from build123d import *

# Parameters (mm, degrees)
BOSS_EXTRUDE1_DEPTH              = 5.334
FILLET1_R                        = 0.508
BOSS_EXTRUDE2_DEPTH              = 1.5875
F_56_0_0465_DIAMETER_HOLE1_D     = 1.1811
F_56_0_0465_DIAMETER_HOLE1_DEPTH = 5.08
CUT_EXTRUDE3_REACH               = 13.094
CUT_EXTRUDE3_START_RADIUS        = 21.519514579
CUT_EXTRUDE3_END_RADIUS          = 21.519514579
SKETCH9_W                        = 0.762
SKETCH9_H                        = 6.35


with BuildPart() as part:
    # Sketch1 → Boss-Extrude1 (new body)
    with BuildSketch(Plane.XY):
        with BuildLine():
            Line((3.301999954, 5.156199954), (-3.301999954, 5.156199954))
            ThreePointArc((-3.301999954, 5.156199954), (-4.613117348, 4.613117348), (-5.156199954, 3.301999954))
            Line((-5.156199954, 3.301999954), (-5.156199954, -3.301999954))
            ThreePointArc((-5.156199954, -3.301999954), (-4.613117348, -4.613117348), (-3.301999954, -5.156199954))
            Line((-3.301999954, -5.156199954), (3.301999954, -5.156199954))
            ThreePointArc((3.301999954, -5.156199954), (4.613117348, -4.613117348), (5.156199954, -3.301999954))
            Line((5.156199954, -3.301999954), (5.156199954, 3.301999954))
            ThreePointArc((5.156199954, 3.301999954), (4.613117348, 4.613117348), (3.301999954, 5.156199954))
        make_face()
    extrude(amount=-BOSS_EXTRUDE1_DEPTH)

    # Fillet1
    fillet1_edges = [part.edges().sort_by_distance(p)[0] for p in [
        (0, 5.156199954, 0),
        (4.613117348, 4.613117348, 0),
        (5.156199954, 0, 0),
        (4.613117348, -4.613117348, 0),
        (0, -5.156199954, 0),
        (-4.613117348, -4.613117348, 0),
        (-5.156199954, 0, 0),
        (-4.613117348, 4.613117348, 0),
    ]]
    fillet(fillet1_edges, radius=FILLET1_R)

    # Sketch4 → Boss-Extrude2 (add)
    with BuildSketch(Plane(origin=(0, 0, -5.334), x_dir=(-1, 0, 0), z_dir=(0, 0, -1))):
        with BuildLine():
            Line((-5.664199954, 3.301999954), (-5.664199954, -3.301999954))
            ThreePointArc((-5.664199954, -3.301999954), (-4.972327592, -4.972327592), (-3.301999954, -5.664199954))
            Line((-3.301999954, -5.664199954), (3.301999954, -5.664199954))
            ThreePointArc((3.301999954, -5.664199954), (4.972327592, -4.972327592), (5.664199954, -3.301999954))
            Line((5.664199954, -3.301999954), (5.664199954, 3.301999954))
            ThreePointArc((5.664199954, 3.301999954), (4.972327592, 4.972327592), (3.301999954, 5.664199954))
            Line((3.301999954, 5.664199954), (-3.301999954, 5.664199954))
            ThreePointArc((-3.301999954, 5.664199954), (-4.972327592, 4.972327592), (-5.664199954, 3.301999954))
        make_face()
    extrude(amount=BOSS_EXTRUDE2_DEPTH)

    # #56 (0.0465) Diameter Hole1
    with Locations(Plane(origin=(0, 0, -6.9215), x_dir=(-1, 0, 0), z_dir=(0, 0, -1))):
        with Locations((0, 0)):
            Hole(F_56_0_0465_DIAMETER_HOLE1_D / 2, depth=F_56_0_0465_DIAMETER_HOLE1_DEPTH)

    # Sketch8 → Cut-Revolve1 (revolve, cut)
    with BuildSketch(Plane(origin=(0, 0, 0), x_dir=(0, 0, -1), z_dir=(1, 0, 0)), mode=Mode.PRIVATE) as cut_revolve1_sk:
        with BuildLine():
            Line((0, 4.648199954), (0, 0))
            Line((0, 0), (0.508, 0))
            ThreePointArc((0.508, 0), (0.380623019, 2.337938558), (0, 4.648199954))
        make_face()
    revolve(cut_revolve1_sk.sketch.rotate(Axis((0, 0, -0.508), (0, 0, 1)), 90), axis=Axis((0, 0, -0.508), (0, 0, 1)), mode=Mode.SUBTRACT)

    # Cut-Extrude3: from a sphere face, 13.094 long prism both ways, kept between that surface and its translate by the depth
    cut_extrude3_start = Location((0, 0, 21.011514579)) * Sphere(CUT_EXTRUDE3_START_RADIUS, mode=Mode.PRIVATE)
    cut_extrude3_end = Location((0, 0, 20.503514579)) * Sphere(CUT_EXTRUDE3_END_RADIUS, mode=Mode.PRIVATE)
    # Sketch9 → Cut-Extrude3 (cut, from a surface)
    with BuildSketch(Plane.XY, mode=Mode.PRIVATE) as cut_extrude3_sk1:
        Rectangle(SKETCH9_W, SKETCH9_H)
    cut_extrude3_tool1 = extrude(cut_extrude3_sk1.sketch, amount=CUT_EXTRUDE3_REACH, both=True, mode=Mode.PRIVATE)
    add(((cut_extrude3_tool1 - cut_extrude3_start) & cut_extrude3_end).solids().sort_by_distance((0, 0, -0.52308))[0], mode=Mode.SUBTRACT)


solid = part.part
Input: part model. Units: mm. Frame: model coordinates. A direction names the side the tool comes from. Coordinates: 2 decimals unless noted, no trailing zeros. Loops run counter-clockwise (first coordinate to the right, second up) from the corner with the lowest first, then second, coordinate; pieces in that order, holes last. Notation, with made-up numbers: (86.25, 52) -> (97.25, 52) arc R12 ccw to (97.25, 63) -> close; hole circle Ø3 at (-8, 33). An arc over 180 degrees is marked (long way). Write item = value, one per line. Start each with the question number.
Item 1: Mould query, pull axis Y, two halves, no side actions, for faces 1 (the face through (0, 0, -1.842)), 2 (the face through (-4, 4, 0)), 3 (the face through (4.954, 4.991, -6.117)), 4 (the face through (-4.954, -4.991, -6.117)). Classes: pulls with the +Y half, pulls with the -Y half, needs draft (parallel to the pull), parting line crosses it, or undercut.
Item 2: First-contact query: P1, Ø2, axis at x = 3.5, z = -5.5, coming from the +Y side; P2, Ø0.6, axis at y = -1, z = -0.5, coming from the +X side; P3, Ø1, axis at y = -4.5, z = -5, coming from the -X side; P4, Ø0.9, axis at x = 0, y = 0, coming from the -Z side. Flat tips, straight axial feed; report the tip coordinate or a pass-through.
Item 3: Reachability of faces 5 (the face through (4.599, -4.627, -2.887)), 6 (the face through (-4.599, 4.627, -2.887)), 7 (the face through (-5.156, 0, -3)), 8 (the face through (4.627, 4.599, -2.887)) from +Z, -Z, +X, -X, +Y, -Y: full face, straight path, thin tool, end or side. Return the list, or none.
Item 4: Material intervals for line 1 (Y direction, x = 0, z = -3.35); line 2 (X direction, y = -2.5, z = -0.5); line 3 (Y direction, x = -0.25, z = -4), sorted ascending.
Item 5: Cut plane C-C, the plane y = 3. Return loops of the section in (x, z).
Item 6: Cut plane A-A, the plane z = -4.75. Return loops of the section in (x, y).
Item 7: Cut plane D-D, the plane z = -5.75. Return loops of the section in (x, y).
Item 8: Cut plane B-B, the plane x = 1. Return loops of the section in (y, z).
Ans:
q1.face_1 = undercut
q1.face_2 = needs draft
q1.face_3 = pulls with the +Y half
q1.face_4 = pulls with the -Y half
q2.P1 = 5.66
q2.P2 = 5.16
q2.P3 = -5.52
q2.P4 = -1.84
q3.face_5 = +Z, +X, -Y
q3.face_6 = +Z, -X, +Y
q3.face_7 = +Z, -X, +Y, -Y
q3.face_8 = +Z, +X, +Y
q4.line_1 = -5.16 to -0.59, 0.59 to 5.16
q4.line_2 = -5.16 to -0.38, 0.38 to 5.16
q4.line_3 = -5.16 to -0.54, 0.54 to 5.16
q5.outline = (-5.66, -6.92) -> (5.66, -6.92) -> (5.66, -5.33) -> (5.16, -5.33) -> (5.16, -0.51) arc R0.51 ccw to (4.65, 0) -> (3.55, 0) arc R21.31 cw to (0.38, -0.29) -> (0.38, -0.8) arc R21.31 cw to (-0.38, -0.8) -> (-0.38, -0.29) arc R21.31 cw to (-3.55, 0) -> (-4.65, 0) arc R0.51 ccw to (-5.16, -0.51) -> (-5.16, -5.33) -> (-5.66, -5.33) -> close
q6.outline = (-5.16, -3.3) arc R1.85 ccw to (-3.3, -5.16) -> (3.3, -5.16) arc R1.85 ccw to (5.16, -3.3) -> (5.16, 3.3) arc R1.85 ccw to (3.3, 5.16) -> (-3.3, 5.16) arc R1.85 ccw to (-5.16, 3.3) -> close; hole circle Ø1.18 at (0, 0)
q7.outline = (-5.66, -3.3) arc R2.36 ccw to (-3.3, -5.66) -> (3.3, -5.66) arc R2.36 ccw to (5.66, -3.3) -> (5.66, 3.3) arc R2.36 ccw to (3.3, 5.66) -> (-3.3, 5.66) arc R2.36 ccw to (-5.66, 3.3) -> close; hole circle Ø1.18 at (0, 0)
q8.outline = (-5.66, -6.92) -> (5.66, -6.92) -> (5.66, -5.33) -> (5.16, -5.33) -> (5.16, -0.51) arc R0.51 ccw to (4.65, 0) -> (4.54, 0) arc R21.5 cw to (-4.54, 0) -> (-4.65, 0) arc R0.51 ccw to (-5.16, -0.51) -> (-5.16, -5.33) -> (-5.66, -5.33) -> close
